Part model, mm, in its own coordinate system. A direction names the side the tool comes from. Round coordinates to 2 decimals unless told otherwise and drop trailing zeros. Write each loop counter-clockwise with the first axis right and the second up, starting at its lowest first coordinate (ties: lowest second). Pieces come first, ordered by that corner, then holes.
1) Drill centre lines: L1, parallel to Y at x = 0, z = 2.15; L2, parallel to Z at x = -11.5, y = 11; L3, parallel to Y at x = 0, z = -4.3. Where is each one in solid material? Low to high.
2) Which spindle directions (+Z, -Z, +X, -X, +Y, -Y) get a long thin tool onto all of the face, cutting with end or side? Do faces 4 (the flat face through (11, 0, 2.5)), 5 (the cylindrical face through (8.69, -6.66, -4.74)). Say none if no direction does.
3) Pull direction X, two halves, no side cores. Call faces 1 (the cylindrical face through (-7.702, 7.063, 1.76)), 2 (the flat face through (-12, -4, -2.5)), 3 (the flat face through (17.5, 0, 0)): +X half, -X half, draft (parallel to the pull), parting line (faces both ways), or undercut.
4) Saw through at D-D on x = 13.5. Write the cut outline in (y, z), and give its area (3 significant figures).
5) Saw through at C-C on z = -3.25. Write the cut outline in (x, y), and give its area (3 significant figures).
```python
from build123d import *

# Parameters (mm, degrees)
SKETCH1_W           = 35
SKETCH1_H           = 40
BOSS_EXTRUDE1_DEPTH = 2.5
SKETCH5_R           = 10.95
BOSS_EXTRUDE2_DEPTH = 3
SKETCH2_R           = 8.95
CUT_EXTRUDE1_DEPTH  = 28.753378173
SKETCH6_R           = 10.45
CUT_EXTRUDE2_DEPTH  = 3
CHAMFER2_SIZE       = 1.5


with BuildPart() as part:
    # Sketch1 → Boss-Extrude1 (new, symmetric)
    with BuildSketch(Plane.XY):
        Rectangle(SKETCH1_W, SKETCH1_H)
    extrude(amount=BOSS_EXTRUDE1_DEPTH, both=True)

    # Sketch5 → Boss-Extrude2 (add)
    with BuildSketch(Plane(origin=(0, 0, -2.5), x_dir=(-1, 0, 0), z_dir=(0, 0, -1))):
        Circle(SKETCH5_R)
    extrude(amount=BOSS_EXTRUDE2_DEPTH)

    # Sketch2 → Cut-Extrude1 (cut, through all)
    with BuildSketch(Plane.XY.offset(2.5)):
        Circle(SKETCH2_R)
    extrude(amount=-CUT_EXTRUDE1_DEPTH, mode=Mode.SUBTRACT)

    # Sketch6 → Cut-Extrude2 (cut)
    with BuildSketch(Plane.XY.offset(2.5)):
        Circle(SKETCH6_R)
    extrude(amount=-CUT_EXTRUDE2_DEPTH, mode=Mode.SUBTRACT)

    # Chamfer2
    chamfer2_edges = [part.edges().sort_by_distance(p)[0] for p in [
        (10.95, 0, -2.5),
        (-10.45, 0, -0.5),
    ]]
    chamfer(chamfer2_edges, length=CHAMFER2_SIZE - 0.0001)  # a hair under: the kernel refuses the full size


solid = part.part
```
Completed:
1. L1: y = -20 to -10.45, 10.45 to 20
1. L2: z = -2.5 to 2.5
1. L3: y = -10.95 to -8.95, 8.95 to 10.95
2. face 4: +Z, +X, -X, +Y, -Y
2. face 5: -Z
3. face 1: undercut
3. face 2: draft
3. face 3: +X half
4. outline: (-20, -2.5) - (20, -2.5) - (20, 2.5) - (-20, 2.5) - close
4. area: 200 mm2
5. outline: circle Ø23.4 at (0, 0); hole circle Ø17.9 at (0, 0)
5. area: 178 mm2
